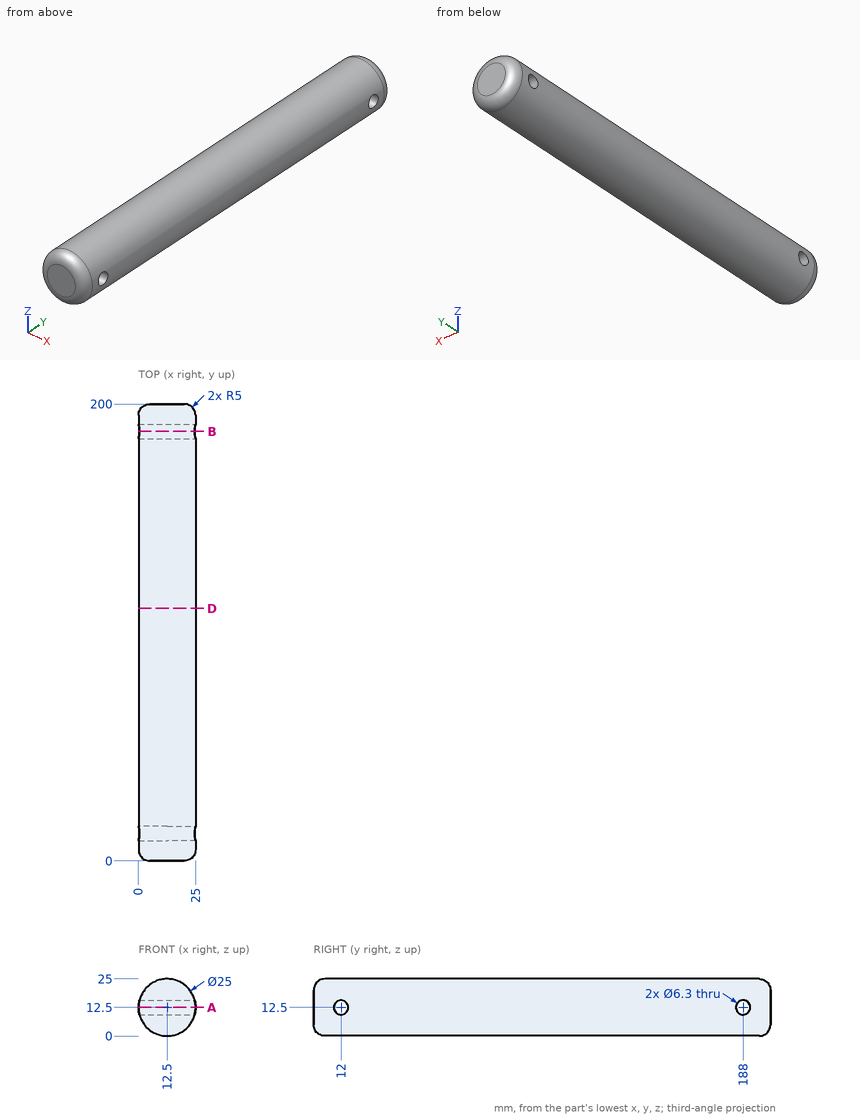
Design review of the part shown in the three views and the two pictorial views. Dimensions are in mm from the part's minimum x, y and z. Round coordinates to 2 decimals unless told otherwise and drop trailing zeros. Write each loop counter-clockwise with the first axis right and the second up, starting at its lowest first coordinate (ties: lowest second). Pieces come first, ordered by that corner, then holes. Notation, with made-up numbers: (-6, 50.5) - (53, 50.5) arc R36 cw to (53, 84.5) - close; hole circle Ø11 at (86.5, 67). An arc over 180 degrees is marked (long way). Write item = value, one per line. Start each with the question number.
1. Consider section B-B on y = 188. State the section outline as (x, z) points.
2. Consider section D-D on y = 110.5. State the section outline as (x, z) points, plus the area to 3 significant figures.
3. Consider section A-A on z = 12.5. Give the number of separate pieces and of enclosed holes in the cut face, plus the area to 3 significant figures.
4. Wall thickness on L1, parallel to Y at x = 1.25, z = 12.75; L2, parallel to Y at x = 10.75, z = 13.5; L3, parallel to Z at x = 18.25, y = 12: over which ranges is each line inside the solid? List them lowest first.
5. For pin 1 Ø6 at (x, y) = (3, 31.5) entering from -Z; pin 2 Ø4 at (y, z) = (136.5, 4) entering from -X; pin 3 Ø6 at (x, y) = (2.5, 71.5) entering from +Z, all flat-tipped, find the tip position at first contact; note any pin that passes through.
Evaluation:
q1.outline = (0.4, 9.35) arc R12.5 ccw to (24.6, 9.35) - close; (0.4, 15.65) - (24.6, 15.65) arc R12.5 ccw to start
q2.outline = circle Ø25 at (12.5, 12.5)
q2.area = 491 mm2
q3.separate_pieces = 3
q3.enclosed_holes = 0
q3.area = 4,660 mm2
q4.L1 = 1.7 to 8.86, 15.14 to 184.86, 191.14 to 198.3
q4.L2 = 0 to 9.01, 14.99 to 185.01, 190.99 to 200
q4.L3 = 1.4 to 9.35, 15.65 to 23.6
q5.pin_1 = 1.82
q5.pin_2 = 1.82
q5.pin_3 = 22.86
